```python
from build123d import *

# Parameters (mm, degrees)
F1_DEPTH = 35
F0_W     = 6
F0_H     = 20
F0_R     = 2.5
F0_W_2   = 30
F2_DEPTH = 5
F3_R     = 2
F4_SIZE  = 3
F5_R     = 1
F6_SIZE  = 2
F7_R     = 2
F9_DEPTH = 12.5


# Not quite as in the source:
# - a fillet or chamfer that OpenCascade refuses, or shapes differently, is made with other operations: its cross-section is extruded or revolved along the edge and cut away or added
# - a feature names something its author has since deleted; it is built from what else it names


with BuildPart() as f1:
    # F0 (on Top) → F1 (new body)
    with BuildSketch(Plane.XY):
        Polygon((-89.3438757165, 20.7090974661), (-89.3438757165, 30.7090974661), (-95.3438757165, 30.7090974661), (-95.3438757165, 10.7090974661), (-89.3438757165, 10.7090974661), align=None)
    extrude(amount=F1_DEPTH)



with BuildPart() as f1b:
    # F0 (on Top) → F1, piece 2 (new body)
    with BuildSketch(Plane.XY):
        with Locations((-48.3438757165, 20.7090974661)):
            Rectangle(F0_W, F0_H)
    extrude(amount=F1_DEPTH)


with BuildPart() as f1_1:
    add(f1.part)

    add(f1b.part)  # F2 merges F1b
    # F0 (on Top) → F2 (join)
    with BuildSketch(Plane.XY):
        Polygon((-51.3438757165, 30.7090974661), (-89.3438757165, 30.7090974661), (-89.3438757165, 20.7090974661), (-89.3438757165, 10.7090974661), (-51.3438757165, 10.7090974661), align=None)
        with Locations((-71.4934170246, 20.7090974661)):
            Circle(F0_R, mode=Mode.SUBTRACT)
        with Locations((-57.2206377983, 20.7090974661)):
            Circle(F0_R, mode=Mode.SUBTRACT)
        with Locations((-30.3438757165, 20.7090974661)):
            Rectangle(F0_W_2, F0_H)
        with Locations((-36.3354164958, 20.7090974661)):
            Circle(F0_R, mode=Mode.SUBTRACT)
        with Locations((-24.3354164958, 20.7090974661)):
            Circle(F0_R, mode=Mode.SUBTRACT)
    extrude(amount=F2_DEPTH)

    # F3
    f3_edges = [f1_1.edges().sort_by_distance(p)[0] for p in [
        (-89.343876, 20.709097, 5),
        (-51.343876, 20.709097, 5),
        (-45.343876, 20.709097, 35),
    ]]
    fillet(f3_edges, radius=F3_R)

    # F4
    f4_edges = [f1_1.edges().sort_by_distance(p)[0] for p in [
        (-15.343876, 20.709097, 0),
    ]]
    chamfer(f4_edges, length=F4_SIZE)

    # F5
    f5_edges = [f1_1.edges().sort_by_distance(p)[0] for p in [
        (-15.343876, 20.709097, 3),
    ]]
    fillet(f5_edges, radius=F5_R)

    # F6
    f6_edges = [f1_1.edges().sort_by_distance(p)[0] for p in [
        (-59.720638, 20.709097, 0),
        (-38.835416, 20.709097, 0),
        (-26.835416, 20.709097, 0),
        (-73.993417, 20.709097, 0),
    ]]
    chamfer(f6_edges, length=F6_SIZE)

    # F7
    f7_edges = [f1_1.edges().sort_by_distance(p)[0] for p in [
        (-95.343876, 20.709097, 35),
        (-95.343876, 20.709097, 0),
    ]]
    fillet(f7_edges, radius=F7_R)

    # F8 (on face) → F9 (cut, symmetric)
    with BuildSketch(Plane(origin=(-95.3438757165, 0, 0), x_dir=(0, -1, 0), z_dir=(-1, 0, 0))):
        with BuildLine():
            ThreePointArc((-18.2090974661, 28.8686309451), (-18.9413305132, 30.636397898), (-20.7090974661, 31.3686309451))
            Line((-20.7090974661, 31.3686309451), (-20.7090974661, 26.3686309451))
            ThreePointArc((-20.7090974661, 26.3686309451), (-18.9413305132, 27.1008639921), (-18.2090974661, 28.8686309451))
        make_face()
        with BuildLine():
            Line((-20.7090974661, 26.3686309451), (-20.7090974661, 31.3686309451))
            ThreePointArc((-20.7090974661, 31.3686309451), (-23.2090974661, 28.8686309451), (-20.7090974661, 26.3686309451))
        make_face()
    extrude(amount=F9_DEPTH, both=True, mode=Mode.SUBTRACT)

    # F10: chamfer of 2 on 1 edges, made by hand

    # F10_s1 → F10_t2 (revolve, cut)
    with BuildSketch(Plane.XY.offset(28.8686309451)):
        Polygon((-95.3438757165, 16.2090974661), (-93.3438757165, 18.2090974661), (-95.3438757165, 18.2090974661), align=None)
    revolve(axis=Axis((-95.3438757165, 20.7090974661, 28.8686309451), (-1, 0, 0)), mode=Mode.SUBTRACT)


solid = f1_1.part
```
CAD build for the part. Positions are in the model's coordinates, mm. A direction names the side the tool comes from. Round coordinates to 2 decimals unless told otherwise and drop trailing zeros. Order: outer loops, then holes, each group sorted by start corner. A loop starts at its lowest first (then second) coordinate and runs counter-clockwise, first axis right, second up. Notation, with made-up numbers: (11.25, 12.5) - (38.25, 12.5) arc R12 cw to (38.25, 18.5) - close; hole circle Ø6 at (80, -36.5). An arc over 180 degrees is marked (long way). Answer in a Markdown table with one row per item. Add a question column.
(1) Band-saw the part on A-A on z = 20. List the corners of the cut face in (x, y).
(2) Probe L1, parallel to X at y = 20, z = 11.5; L2, parallel to Z at x = -56.5, y = 14; L3, parallel to Z at x = -91, y = 21.5. List the from-to ranges inside material, lowest first. Write a range as [from, to].
(3) 3-axis set-ups, long thin cutter, end or side, ignore diameter. For faces 4 (the face through (-95.344, 21, 17)), 5 (the face through (-88.77, 20.57, 5.6)): which of +Z, -Z, +X, -X, +Y, -Y reach the whole face in a straight line?
(4) Band-saw the part on D-D on x = -82. List the corners of the cut face in (y, z), and give its area (3 significant figures).
(5) Mould opens along Y. For faces 1 (the face through (-70.34, 18.49, 3.48)), 2 (the face through (-64, 10.709, 4)), 3 (the face through (-56.4, 25.3, 0)) say: +Y half, -Y half, draft (parallel to the pull), parting line (faces both ways), or undercut.
(6) Band-saw the part on B-B on y = 14.25. List the corners of the cut face in (x, z), and give its area (3 significant figures).
(7) Band-saw the part on C-C on z = 6. List the corners of the cut face in (x, y), and give its area (3 significant figures).
(8) Drop flat-ended pins along their axis: pin 1 Ø6.5 at (x, y) = (-24.34, 20.71) entering from -Z; pin 2 Ø10 at (x, y) = (-37.5, 23.5) entering from +Z; pin 3 Ø8 at (x, y) = (-57.22, 20.71) entering from -Z. Give the stop position or say it passes through.
Data:
| question | item | result |
|---|---|---|
| 1 | outline | (-95.34, 10.71) - (-89.34, 10.71) - (-89.34, 30.71) - (-95.34, 30.71) - close; (-51.34, 10.71) - (-45.34, 10.71) - (-45.34, 30.71) - (-51.34, 30.71) - close |
| 2 | L1 | x = [-95.34, -89.34], [-51.34, -45.34] |
| 2 | L2 | z = [0, 5] |
| 2 | L3 | z = [0, 26.5], [31.24, 35] |
| 3 | face 4 | +Z, -Z, -X, +Y, -Y |
| 3 | face 5 | +Z, +Y, -Y |
| 4 | outline | (10.71, 0) - (30.71, 0) - (30.71, 5) - (10.71, 5) - close |
| 4 | area | 100 mm^2 |
| 5 | face 1 | undercut |
| 5 | face 2 | -Y half |
| 5 | face 3 | draft |
| 6 | outline | (-95.34, 2) arc R2 ccw to (-93.34, 0) - (-18.34, 0) - (-15.64, 2.71) arc R1 ccw to (-15.34, 3.41) - (-15.34, 5) - (-45.34, 5) - (-45.34, 33) arc R2 ccw to (-47.34, 35) - (-51.34, 35) - (-51.34, 7) arc R2 cw to (-53.34, 5) - (-87.34, 5) arc R2 cw to (-89.34, 7) - (-89.34, 35) - (-93.34, 35) arc R2 ccw to (-95.34, 33) - close |
| 6 | area | 755 mm^2 |
| 7 | outline | (-95.34, 10.71) - (-89.08, 10.71) - (-89.08, 30.71) - (-95.34, 30.71) - close; (-51.61, 10.71) - (-45.34, 10.71) - (-45.34, 30.71) - (-51.61, 30.71) - close |
| 7 | area | 251 mm^2 |
| 8 | pin 1 | stops at z = 1.25 |
| 8 | pin 2 | stops at z = 5 |
| 8 | pin 3 | stops at z = 0.5 |
